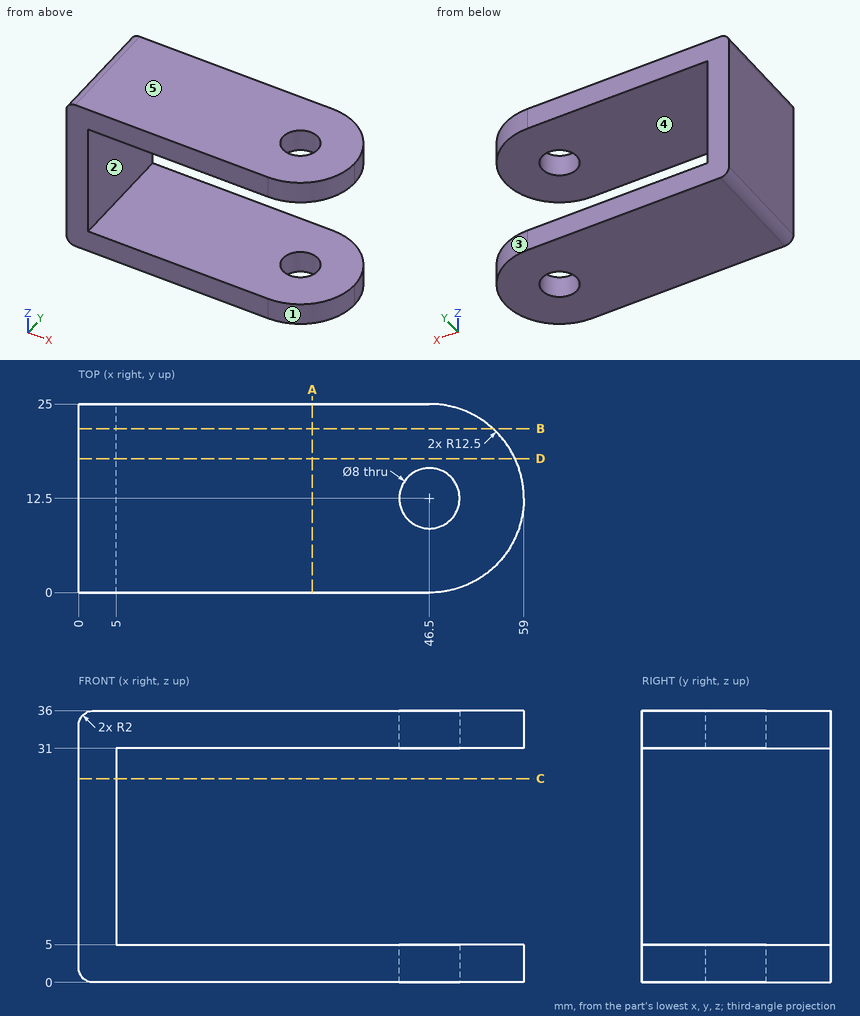
Can you work these out from the drawing? Everything is in mm from the part's minimum corner. A direction names the side the tool comes from. Give positions to 0.01 mm unless a question says otherwise; leave off trailing zeros. Order: outer loops, then holes, each group sorted by start corner. A loop starts at its lowest first (then second) coordinate and runs counter-clockwise, first axis right, second up. Notation, with made-up numbers: M 84,73 L 139,73 A23 cw 139,95 Z; hole C 14.5,7.5 d4. An arc over 180 degrees is marked long. Use a Markdown table: item, result. Add a question column.
Item 1: Suppose I cut it at D-D (y = 17.75). List the corners of the cut face in (x, z) for me.
Item 2: We'd pull the mould along Z, two halves only. Please class the marked faces 3, 4 and 5: +Z half, -Z half, draft (parallel to the pull), parting line (faces both ways), or undercut.
Item 3: For the marked faces 1 and 2, which set-ups out of +Z, -Z, +X, -X, +Y, -Y let a thin tool reach every point of the face, with its end or its side?
Item 4: Will these pins go through, and if not, where does the flat tip stop? pin 1 (1 mm diameter, centred on y = 19.5, z = 18.5, fed in from +X); pin 2 (5 mm diameter, centred on x = 46.5, y = 12.5, fed in from +Z).
Item 5: Suppose I cut it at A-A (x = 31). List the corners of the cut face in (y, z) for me.
Item 6: Suppose I cut it at C-C (z = 27). List the corners of the cut face in (x, y) for me.
Item 7: Suppose I cut it at B-B (y = 21.75). List the corners of the cut face in (x, z) for me.
Item 8: If I drill on L1, parallel to Z at x = 25, y = 7.25; L2, parallel to Y at x = 46.5, z = 2.7; L3, parallel to X at y = 12.25, z = 32.5, over which ranges is the centre line in solid material (lowest first)? Write a range as [from, to].
Answer sheet:
| question | item | result |
|---|---|---|
| 1 | outline | M 0,2 A2 ccw 2,0 L 57.84,0 L 57.84,5 L 5,5 L 5,31 L 57.84,31 L 57.84,36 L 2,36 A2 ccw 0,34 Z |
| 2 | face 3 | draft |
| 2 | face 4 | undercut |
| 2 | face 5 | +Z half |
| 3 | face 1 | +Z, -Z, +X, -Y |
| 3 | face 2 | +X, +Y, -Y |
| 4 | pin 1 | stops at x = 5 |
| 4 | pin 2 | passes through |
| 5 | outline | M 0,0 L 25,0 L 25,5 L 0,5 Z; M 0,31 L 25,31 L 25,36 L 0,36 Z |
| 6 | outline | M 0,0 L 5,0 L 5,25 L 0,25 Z |
| 7 | outline | M 0,2 A2 ccw 2,0 L 54.91,0 L 54.91,5 L 5,5 L 5,31 L 54.91,31 L 54.91,36 L 2,36 A2 ccw 0,34 Z |
| 8 | L1 | z = [0, 5], [31, 36] |
| 8 | L2 | y = [0, 8.5], [16.5, 25] |
| 8 | L3 | x = [0, 42.51], [50.49, 59] |
